Geometry: final body of the model. Coordinates: model frame, mm. Face numbers are marked on the shaded views. A direction names the side the tool comes from. Give positions to 0.01 mm unless a question says otherwise; leave off trailing zeros. Write each loop counter-clockwise with the first axis right and the second up, starting at its lowest first coordinate (ties: lowest second). Pieces come first, ordered by that corner, then holes.
Q1. Section C-C (y = 17.5). Return the cut outline in (x, z).
Q2. Section B-B (z = 15). Return the cut outline in (x, y).
Q3. Reachability of the marked faces 4, 5, 6 and 7 from +Z, -Z, +X, -X, +Y, -Y: full face, straight path, thin tool, end or side. Return the list, or none.
Q4. Mould query, pull axis Z, two halves, no side actions, for the marked faces 1, 2 and 3. Classes: +Z half, -Z half, draft (parallel to the pull), parting line (faces both ways), or undercut.
Q5. Section A-A (y = -1). Return the cut outline in (x, z).
Q6. Pin query (flat end, axial travel): pin 1 Ø12 at (y, z) = (10.5, 17) entering from -X; pin 2 Ø5.5 at (x, y) = (2, 0) entering from +Z; pin 3 Ø2.5 at (x, y) = (0, 7.02) entering from -Z; pin 4 Ø9 at (x, z) = (7, 30.5) entering from +Y. Return the tip coordinate at first contact, or that it passes through.
Q7. Line query: line 1 (Z direction, x = 5, y = 9); line 2 (Y direction, x = 0, z = 1); line 3 (Y direction, x = 0.25, z = 25.5). Output: solid intervals per line, ascending.
Q8. Section D-D (y = 22.27). Return the cut outline in (x, z), plus the area to 3 significant figures.
from build123d import *

# Parameters (mm, degrees)
SKETCH1_W            = 30
SKETCH1_H            = 40
BOSS_EXTRUDE1_DEPTH  = 40
CUT_EXTRUDE1_DEPTH   = 35
SKETCH4_W            = 25
SKETCH4_H            = 35
CUT_EXTRUDE3_DEPTH   = 20
SKETCH5_W            = 25
SKETCH5_H            = 17.5
CUT_EXTRUDE4_DEPTH   = 20
SKETCH13_W           = 25
SKETCH13_H           = 5
BOSS_EXTRUDE3_DEPTH  = 20
CUT_EXTRUDE5_DEPTH   = 40
CUT_EXTRUDE6_START   = -40
CUT_EXTRUDE6_DEPTH   = 40
CUT_EXTRUDE9_START   = -40
SKETCH10_W           = 30
SKETCH10_H           = 10
CUT_EXTRUDE9_DEPTH   = 40
CHAMFER2_SIZE        = 3
CUT_EXTRUDE10_DEPTH  = 28.5
SKETCH17_W           = 25
SKETCH17_H           = 2.5
BOSS_EXTRUDE4_DEPTH  = 10
CUT_EXTRUDE13_START  = -30
SKETCH18_W           = 20
SKETCH18_H           = 3
CUT_EXTRUDE13_DEPTH  = 30
SKETCH19_W           = 16.5
SKETCH19_H           = 6
CUT_EXTRUDE14_DEPTH  = 10
BOSS_EXTRUDE5_DEPTH  = 8.5
SKETCH22_W           = 25
SKETCH22_H           = 5
BOSS_EXTRUDE6_DEPTH  = 1
SKETCH23_W           = 13.292868742
SKETCH23_H           = 5
BOSS_EXTRUDE7_DEPTH  = 15
CHAMFER4_SIZE        = 5
CHAMFER6_SIZE        = 5
SKETCH30_W           = 1.5
SKETCH30_H           = 10
BOSS_EXTRUDE8_DEPTH  = 20
CHAMFER10_SIZE       = 14
CUT_EXTRUDE15_DEPTH  = 25
CHAMFER11_SIZE       = 2
BOSS_EXTRUDE9_START  = 0.75
SKETCH31_R           = 2
BOSS_EXTRUDE9_DEPTH  = 0.75
CHAMFER12_SIZE       = 0.5
CHAMFER13_SIZE       = 0.5
CHAMFER14_SIZE       = 0.75
CHAMFER15_SIZE       = 0.5
BOSS_EXTRUDE10_START = 2
SKETCH32_W           = 3.292868742
SKETCH32_H           = 5.46
BOSS_EXTRUDE10_DEPTH = 2
CHAMFER16_SIZE       = 3
CHAMFER17_SIZE       = 1.5


# Some blends are built 0.0001 mm under size
with BuildPart() as part:
    # Sketch1 → Boss-Extrude1 (new body)
    with BuildSketch(Plane.XY):
        Rectangle(SKETCH1_W, SKETCH1_H)
    extrude(amount=BOSS_EXTRUDE1_DEPTH)

    # Sketch2 → Cut-Extrude1 (cut)
    with BuildSketch(Plane.XY.offset(40)):
        with BuildLine():
            Line((-6.986594306, -2.5), (6.986594306, -2.5))
            ThreePointArc((6.986594306, -2.5), (10.247468698, -10.227783409), (6.646434371, -17.80303852))
            Line((6.646434371, -17.80303852), (-6.646434371, -17.80303852))
            ThreePointArc((-6.646434371, -17.80303852), (-10.247468698, -10.227783409), (-6.986594306, -2.5))
        make_face()
    extrude(amount=-CUT_EXTRUDE1_DEPTH, mode=Mode.SUBTRACT)

    # Sketch4 → Cut-Extrude3 (cut)
    with BuildSketch(Plane(origin=(0, 20, 0), x_dir=(1, 0, 0), z_dir=(0, 1, 0))):
        with Locations((0, -20)):
            Rectangle(SKETCH4_W, SKETCH4_H)
    extrude(amount=-CUT_EXTRUDE3_DEPTH, mode=Mode.SUBTRACT)

    # Sketch5 → Cut-Extrude4 (cut)
    with BuildSketch(Plane(origin=(0, 0, 0), x_dir=(1, 0, 0), z_dir=(0, 1, 0))):
        with Locations((0, -11.25)):
            Rectangle(SKETCH5_W, SKETCH5_H)
    extrude(amount=-CUT_EXTRUDE4_DEPTH, mode=Mode.SUBTRACT)

    # Sketch13 → Boss-Extrude3 (add)
    with BuildSketch(Plane(origin=(0, 0, 0), x_dir=(1, 0, 0), z_dir=(0, 1, 0))):
        with Locations((0, -22.5)):
            Rectangle(SKETCH13_W, SKETCH13_H)
    extrude(amount=BOSS_EXTRUDE3_DEPTH)

    # Sketch8 → Cut-Extrude5 (cut)
    with BuildSketch(Plane.XY.offset(40)):
        with BuildLine():
            Line((-0.546667462, -9.162650201), (0.546667462, -9.162650201))
            ThreePointArc((0.546667462, -9.162650201), (0, -11.425011068), (-0.546667462, -9.162650201))
        make_face()
    extrude(amount=-CUT_EXTRUDE5_DEPTH, mode=Mode.SUBTRACT)

    # Sketch9 → Cut-Extrude6 (cut)
    with BuildSketch(Plane(origin=(0, 0, 0), x_dir=(-1, 0, 0), z_dir=(0, 0, -1)).offset(CUT_EXTRUDE6_START)):
        with BuildLine():
            Line((-0.354264308, 7.849559809), (0.354264308, 7.849559809))
            ThreePointArc((0.354264308, 7.849559809), (0, 6.122216591), (-0.354264308, 7.849559809))
        make_face()
    extrude(amount=CUT_EXTRUDE6_DEPTH, mode=Mode.SUBTRACT)

    # Sketch10 → Cut-Extrude9 (cut)
    with BuildSketch(Plane.XY.offset(40).offset(CUT_EXTRUDE9_START)):
        with Locations((0, 15)):
            Rectangle(SKETCH10_W, SKETCH10_H)
    extrude(amount=CUT_EXTRUDE9_DEPTH, mode=Mode.SUBTRACT)

    # Chamfer2
    chamfer2_edges = [part.edges().sort_by_distance(p)[0] for p in [
        (-15, -5, 0),
        (-15, -5, 40),
        (15, -5, 40),
        (15, -5, 0),
    ]]
    chamfer(chamfer2_edges, length=CHAMFER2_SIZE)

    # Sketch16 → Cut-Extrude10 (cut, symmetric)
    with BuildSketch(Plane(origin=(-12.5, 0, 0), x_dir=(0, 0, -1), z_dir=(1, 0, 0))):
        Polygon((-2.5, 10), (-9.536752506, 10), (-10.366434052, 10), (-10.366434052, -3.164876481), (-9.536752506, -3.164876481), (-2.5, -3.164876481), align=None)
    extrude(amount=CUT_EXTRUDE10_DEPTH, both=True, mode=Mode.SUBTRACT)

    # Sketch17 → Boss-Extrude4 (add)
    with BuildSketch(Plane(origin=(0, 10, 0), x_dir=(1, 0, 0), z_dir=(0, 1, 0))):
        with Locations((0, -36.25)):
            Rectangle(SKETCH17_W, SKETCH17_H)
    extrude(amount=-BOSS_EXTRUDE4_DEPTH)

    # Sketch18 → Cut-Extrude13 (cut)
    with BuildSketch(Plane(origin=(0, 10, 0), x_dir=(1, 0, 0), z_dir=(0, 1, 0)).offset(CUT_EXTRUDE13_START)):
        with Locations((0, -38.5)):
            Rectangle(SKETCH18_W, SKETCH18_H)
    extrude(amount=CUT_EXTRUDE13_DEPTH, mode=Mode.SUBTRACT)

    # Sketch19 → Cut-Extrude14 (cut)
    with BuildSketch(Plane.XZ.offset(20)):
        with Locations((0, 34)):
            Rectangle(SKETCH19_W, SKETCH19_H)
    extrude(amount=-CUT_EXTRUDE14_DEPTH, mode=Mode.SUBTRACT)

    # Sketch20 → Boss-Extrude5 (add)
    with BuildSketch(Plane(origin=(0, 0, 20), x_dir=(-1, 0, 0), z_dir=(0, 0, -1))):
        with BuildLine():
            Line((12.5, -10), (10.25, -10))
            ThreePointArc((10.25, -10), (9.305601869, -14.297472961), (6.646434371, -17.80303852))
            Line((6.646434371, -17.80303852), (-6.646434371, -17.80303852))
            ThreePointArc((-6.646434371, -17.80303852), (-9.305601869, -14.297472961), (-10.25, -10))
            Line((-10.25, -10), (-12.5, -10))
            Line((-12.5, -10), (-12.5, -20))
            Line((-12.5, -20), (12.5, -20))
            Line((12.5, -20), (12.5, -10))
        make_face()
    extrude(amount=BOSS_EXTRUDE5_DEPTH)

    # Sketch22 → Boss-Extrude6 (add)
    with BuildSketch(Plane(origin=(0, 0, 11.5), x_dir=(-1, 0, 0), z_dir=(0, 0, -1))):
        with Locations((0, -17.5)):
            Rectangle(SKETCH22_W, SKETCH22_H)
    extrude(amount=BOSS_EXTRUDE6_DEPTH)

    # Sketch23 → Boss-Extrude7 (add)
    with BuildSketch(Plane(origin=(0, 10, 0), x_dir=(1, 0, 0), z_dir=(0, 1, 0))):
        with Locations((0, -22.5)):
            Rectangle(SKETCH23_W, SKETCH23_H)
        Polygon((6.646434371, 0), (6.646434371, -2.5), (0, -2.5), (-6.646434371, -2.5), (-6.646434371, 0), align=None)
    extrude(amount=BOSS_EXTRUDE7_DEPTH)

    # Chamfer4
    chamfer4_edges = [part.edges().sort_by_distance(p)[0] for p in [
        (6.646434371, 10, 22.5),
        (-6.646434371, 10, 22.5),
        (6.646434371, 10, 1.25),
        (-6.646434371, 10, 1.25),
    ]]
    chamfer(chamfer4_edges, length=CHAMFER4_SIZE)

    # Chamfer6
    chamfer6_edges = [part.edges().sort_by_distance(p)[0] for p in [
        (6.646434371, 25, 22.5),
        (-6.646434371, 25, 22.5),
        (6.646434371, 25, 1.25),
        (-6.646434371, 25, 1.25),
    ]]
    chamfer(chamfer6_edges, length=CHAMFER6_SIZE)

    # Sketch30 → Boss-Extrude8 (add)
    with BuildSketch(Plane(origin=(0, 0, 0), x_dir=(1, 0, 0), z_dir=(0, 1, 0))):
        with Locations((-5.896434371, -30)):
            Rectangle(SKETCH30_W, SKETCH30_H)
        with Locations((5.896434371, -30)):
            Rectangle(SKETCH30_W, SKETCH30_H)
    extrude(amount=BOSS_EXTRUDE8_DEPTH)

    # Chamfer10
    # the kernel refuses this chamfer: 14 mm, written as the material it takes off along each edge
    with BuildSketch(Plane(origin=(-30.85712746, 20, 35), x_dir=(0, -0.9996219169112968, 0.02749587661058661), z_dir=(1, 0, 0))) as chamfer10_piece_1_section:
        Polygon((CHAMFER10_SIZE * 0.999621916911, CHAMFER10_SIZE * 0.0274958766106), (-CHAMFER10_SIZE * 0.0274958766106, CHAMFER10_SIZE * 0.999621916911), (0, 0), align=None)
    chamfer10_piece_1 = extrude(amount=73.507123663, mode=Mode.PRIVATE)
    chamfer10_piece_1 = split(chamfer10_piece_1, bisect_by=Plane(origin=(5.896434371, 10, 30.768271906), z_dir=(0, 1, 0)), keep=Keep.TOP, mode=Mode.PRIVATE)
    chamfer10_piece_1 = split(chamfer10_piece_1, bisect_by=Plane(origin=(5.896434371, 15.768271906, 25), z_dir=(0, 0, 1)), keep=Keep.TOP, mode=Mode.PRIVATE)
    add(chamfer10_piece_1, mode=Mode.SUBTRACT)
    with BuildSketch(Plane(origin=(30.85712746, 20, 35), x_dir=(0, -0.9996219169112968, 0.02749587661058661), z_dir=(-1, 0, 0))) as chamfer10_piece_2_section:
        Polygon((CHAMFER10_SIZE * 0.999621916911, -CHAMFER10_SIZE * 0.0274958766106), (-CHAMFER10_SIZE * 0.0274958766106, -CHAMFER10_SIZE * 0.999621916911), (0, 0), align=None)
    chamfer10_piece_2 = extrude(amount=73.507123663, mode=Mode.PRIVATE)
    chamfer10_piece_2 = split(chamfer10_piece_2, bisect_by=Plane(origin=(-5.896434371, 10, 30.768271906), z_dir=(0, 1, 0)), keep=Keep.TOP, mode=Mode.PRIVATE)
    chamfer10_piece_2 = split(chamfer10_piece_2, bisect_by=Plane(origin=(-5.896434371, 15.768271906, 25), z_dir=(0, 0, 1)), keep=Keep.TOP, mode=Mode.PRIVATE)
    add(chamfer10_piece_2, mode=Mode.SUBTRACT)

    # Sketch29 → Cut-Extrude15 (cut)
    with BuildSketch(Plane(origin=(0, 0, 0), x_dir=(-1, 0, 0), z_dir=(0, 0, -1))):
        with BuildLine():
            Line((-0.403434811, 23.074512494), (0.403434811, 23.074512494))
            ThreePointArc((0.403434811, 23.074512494), (0, 21.37), (-0.403434811, 23.074512494))
        make_face()
    extrude(amount=-CUT_EXTRUDE15_DEPTH, mode=Mode.SUBTRACT)

    # Chamfer11
    chamfer11_edges = [part.edges().sort_by_distance(p)[0] for p in [
        (12.5, -11.58243824, 2.5),
        (-12.5, -11.58243824, 2.5),
    ]]
    chamfer(chamfer11_edges, length=CHAMFER11_SIZE)

    # Sketch31 → Boss-Extrude9 (add)
    with BuildSketch(Plane.XY.offset(2.5).offset(BOSS_EXTRUDE9_START)):
        with Locations(Location((0, 7.022216591, 0), (0, 0, 180))):
            Circle(SKETCH31_R)
        with BuildLine():
            Line((-0.354264308, 7.849559809), (0.354264308, 7.849559809))
            ThreePointArc((0.354264308, 7.849559809), (0, 6.122216591), (-0.354264308, 7.849559809))
        make_face(mode=Mode.SUBTRACT)
    extrude(amount=-BOSS_EXTRUDE9_DEPTH)

    # Chamfer12
    chamfer12_edges = [part.edges().sort_by_distance(p)[0] for p in [
        (0, 6.122216591, 3.25),
    ]]
    chamfer(chamfer12_edges, length=CHAMFER12_SIZE)

    # Chamfer13
    chamfer13_edges = [part.edges().sort_by_distance(p)[0] for p in [
        (0, 7.849559809, 3.25),
    ]]
    chamfer(chamfer13_edges, length=CHAMFER13_SIZE)

    # Chamfer14
    chamfer14_edges = [part.edges().sort_by_distance(p)[0] for p in [
        (2, 7.022216591, 2.5),
    ]]
    chamfer(chamfer14_edges, length=CHAMFER14_SIZE - 0.0001)  # a hair under: the kernel refuses the full size

    # Chamfer15
    chamfer15_edges = [part.edges().sort_by_distance(p)[0] for p in [
        (0, 21.37, 25),
        (0, 23.074512494, 25),
        (0, 7.849559809, 25),
        (0, 6.122216591, 25),
    ]]
    chamfer(chamfer15_edges, length=CHAMFER15_SIZE)

    # Sketch32 → Boss-Extrude10 (add)
    with BuildSketch(Plane(origin=(0, 0, 0), x_dir=(-1, 0, 0), z_dir=(0, 0, -1)).offset(BOSS_EXTRUDE10_START)):
        with Locations((0, 22.27)):
            Rectangle(SKETCH32_W, SKETCH32_H)
        with BuildLine():
            Line((0.403434811, 23.074512494), (-0.403434811, 23.074512494))
            ThreePointArc((-0.403434811, 23.074512494), (0, 21.37), (0.403434811, 23.074512494))
        make_face(mode=Mode.SUBTRACT)
    extrude(amount=-BOSS_EXTRUDE10_DEPTH)

    # Chamfer16
    # the kernel refuses this chamfer: 3 mm, written as the material it adds along each edge
    with BuildSketch(Plane(origin=(1.646434371, 19.54, 0), x_dir=(0, -0.9996219169112968, 0.02749587661058636), z_dir=(-1, 0, 0))) as chamfer16_piece_1_section:
        Polygon((CHAMFER16_SIZE * 0.999621916911, -CHAMFER16_SIZE * 0.0274958766106), (-CHAMFER16_SIZE * 0.0274958766106, -CHAMFER16_SIZE * 0.999621916911), (0, 0), align=None)
    chamfer16_piece_1 = extrude(amount=3.292868742, mode=Mode.PRIVATE)
    chamfer16_piece_1 = split(chamfer16_piece_1, bisect_by=Plane(origin=(0, 18.447908995, -2), z_dir=(0, 0, 1)), keep=Keep.TOP, mode=Mode.PRIVATE)
    add(chamfer16_piece_1)

    # Chamfer17
    chamfer17_edges = [part.edges().sort_by_distance(p)[0] for p in [
        (0, 25, -2),
    ]]
    chamfer(chamfer17_edges, length=CHAMFER17_SIZE)


solid = part.part
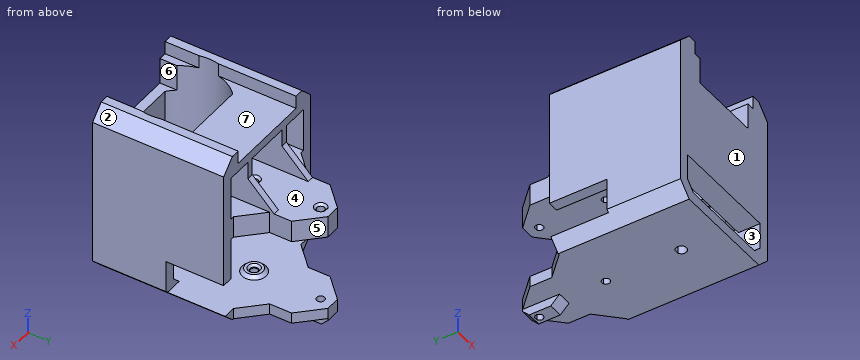
Computed:
1. outline: (-6.65, 0) - (-1.65, 0) - (-1.65, -0.96) - (1.65, -0.96) - (1.65, 0) - (6.65, 0) - (6.65, 2.5) - (-6.65, 2.5) - close; (-6.65, 20) - (6.65, 20) - (6.65, 25) - (-6.65, 25) - close
2. outline: (-15, -20) - (15, -20) - (15, 10) - (12.5, 10) - (12.5, -10) - (10.25, -10) arc R10.25 cw to (6.65, -17.8) - (-6.65, -17.8) arc R10.25 cw to (-10.25, -10) - (-12.5, -10) - (-12.5, 10) - (-15, 10) - close
3. face 4: +Y
3. face 5: +Z, -Z, +X, +Y
3. face 6: +Z, -Y
3. face 7: +Z, +Y, -Y
4. face 1: draft
4. face 2: +Z half
4. face 3: undercut
5. outline: (-15, 10.37) - (-12.5, 10.37) - (-12.5, 20) - (12.5, 20) - (12.5, 10.37) - (15, 10.37) - (15, 37) - (12, 40) - (10, 40) - (10, 37) - (-10, 37) - (-10, 40) - (-12, 40) - (-15, 37) - close; (-14.5, 2.5) - (-12, 0) - (12, 0) - (14.5, 2.5) - close
6. pin 1: stops at x = -15
6. pin 2: stops at z = 37
6. pin 3: stops at z = 0
6. pin 4: stops at y = 14.99
7. line 1: z = 0 to 2.5, 20 to 25, 35 to 37
7. line 2: y = -20 to -11.43, -9.16 to 6.12, 7.85 to 21.37, 23.07 to 25
7. line 3: y = -20 to -17.8, -2.5 to 0
8. outline: (-4.38, 0) - (-1.65, 0) - (-1.65, -2) - (-0.9, -2) - (-0.9, 2.5) - (-4.38, 2.5) - close; (-4.38, 20) - (-0.9, 20) - (-0.9, 24.5) - (-1.4, 25) - (-4.38, 25) - close; (0.9, -2) - (1.65, -2) - (1.65, 0) - (4.38, 0) - (4.38, 2.5) - (0.9, 2.5) - close; (0.9, 20) - (4.38, 20) - (4.38, 25) - (1.4, 25) - (0.9, 24.5) - close
8. area: 54.9 mm2
